```python
from build123d import *

# Parameters (mm, degrees)
SKETCH141_R  = 1.8
SKETCH141_W  = 2.5
SKETCH141_H  = 13
PAD112_DEPTH = 3


with BuildPart() as motorcageendcap:
    # Sketch141 → Pad112 (new body)
    with BuildSketch(Plane.XZ.offset(-90)):
        with BuildLine():
            Line((-29.490381, 15), (-39.5, 9.220944))
            Line((-39.5, 9.220944), (-39.5, -9.220944))
            Line((-39.5, -9.220944), (-29.490381, -15))
            Line((-24, -11.830127), (-29.490381, -15))
            Line((-24, -11.830127), (-18.128421, -22))
            Line((-18.128421, -22), (0, -22))
            Line((0, -22), (0, -19))
            ThreePointArc((0, 19), (-19, 0), (0, -19))
            Line((0, 24), (0, 19))
            Line((-16.973721, 24), (0, 24))
            Line((-24, 11.830127), (-16.973721, 24))
            Line((-29.490381, 15), (-24, 11.830127))
        make_face()
        with Locations((-29, 10)):
            Circle(SKETCH141_R, mode=Mode.SUBTRACT)
        with Locations((-29, -10)):
            Circle(SKETCH141_R, mode=Mode.SUBTRACT)
        with Locations((-12, 20)):
            Circle(SKETCH141_R, mode=Mode.SUBTRACT)
        with Locations((-36, 0)):
            Circle(SKETCH141_R, mode=Mode.SUBTRACT)
        with Locations((-30.25, 0)):
            Rectangle(SKETCH141_W, SKETCH141_H, mode=Mode.SUBTRACT)
    extrude(amount=-PAD112_DEPTH)


with BuildPart() as fusion004020018:
    # Part__Mirroring007: instance of MotorCageEndCap
    add(motorcageendcap.part.mirror(Plane(origin=(0, 0, 0), x_dir=(0, -1, 0), z_dir=(1, 0, 0))))

    # Fusion004020018: union MotorCageEndCap
    add(motorcageendcap.part)


solid = fusion004020018.part
```
Can you work these out from the model? Positions are in its coordinate system, mm. A direction names the side the tool comes from. Coordinates: 2 decimals unless noted, no trailing zeros. Loops run counter-clockwise (first coordinate to the right, second up) from the corner with the lowest first, then second, coordinate; pieces in that order, holes last. Notation, with made-up numbers: M 45.5,67.5 L 60.5,67.5 A26 ccw 60.5,100.5 Z; hole C 39,38 d7. An arc over 180 degrees is marked long. Put each result on its own line as item: value. Start each with the question number.
(1) Imagine slicing it at B-B on z = 10. List the corners of the cut face in (x, y) for me, and give its area (3 significant figures).
(2) Which directions (+Z, -Z, +X, -X, +Y, -Y) give clear straight access to the entire face, cutting with the end or side of a thin tool? Please do faces 1 (the face through (-30, 91, -6.5)), 2 (the face through (-34.43, 91.48, 12.15)), 3 (the face through (-26.784, 91.479, 13.437)), 4 (the face through (21.105, 91.479, -16.844)), 5 (the face through (-9, 93, 17)).
(3) Imagine slicing it at D-D on x = 12.5. List the corners of the cut face in (y, z) for me.
(4) Imagine slicing it at C-C on x = -8. List the corners of the cut face in (y, z) for me, and give its area (3 significant figures).
(5) I need wall thicknesses on probe 1 along Z at (x, y) = (-28, 92.85); probe 2 along X at (y, z) = (91.5, 12); probe 3 along X at (y, z) = (90.6, 3.5). Which ranges of each line are inside material? Lowest first, please.
(6) Will these pins go through, and if not, where does the flat tip stop? pin 1 Ø2 at (x, z) = (36, 0) entering from -Y; pin 2 Ø0.8 at (x, y) = (-29.5, 92) entering from -Z; pin 3 Ø1.2 at (x, y) = (30.5, 92) entering from -Z.
(7) Imagine slicing it at A-A on y = 92.15. Give the number of separate pieces and of enclosed holes in the cut face, and give its area (3 significant figures).
(8) We'd pull the mould along X, two halves only. Please class faces 6 (the face through (29, 91, 0)), 7 (the face through (0, 91, -22)), 8 (the face through (-20.536, 91.479, 17.83)), 9 (the face through (-39.5, 91, 0)): +X half, -X half, draft (parallel to the pull), parting line (faces both ways), or undercut.
Worked answers:
1. outline: M -38.15,90 L -30.8,90 L -30.8,93 L -38.15,93 Z; M -27.2,90 L -16.16,90 L -16.16,93 L -27.2,93 Z; M 16.16,90 L 27.2,90 L 27.2,93 L 16.16,93 Z; M 30.8,90 L 38.15,90 L 38.15,93 L 30.8,93 Z
1. area: 110 mm2
2. face 1: +Y, -Y
2. face 2: +Z, -X, +Y, -Y
2. face 3: +Z, +Y, -Y
2. face 4: -Z, +Y, -Y
2. face 5: +Z, -Z, +X, -X, +Y
3. outline: M 90,-22 L 93,-22 L 93,-14.31 L 90,-14.31 Z; M 90,14.31 L 93,14.31 L 93,18.27 L 90,18.27 Z; M 90,21.73 L 93,21.73 L 93,24 L 90,24 Z
4. outline: M 90,-22 L 93,-22 L 93,-17.23 L 90,-17.23 Z; M 90,17.23 L 93,17.23 L 93,24 L 90,24 Z
4. area: 34.6 mm2
5. probe 1: z = -14.14 to -11.5, -8.5 to 8.5, 11.5 to 14.14
5. probe 2: x = -34.69 to -24.29, -23.9 to -14.73, 14.73 to 23.9, 24.29 to 34.69
5. probe 3: x = -39.5 to -31.5, -29 to -18.67, 18.67 to 29, 31.5 to 39.5
6. pin 1: passes through
6. pin 2: stops at z = -15
6. pin 3: stops at z = -14.76
7. separate pieces: 1
7. enclosed holes: 11
7. area: 1,560 mm2
8. face 6: undercut
8. face 7: draft
8. face 8: undercut
8. face 9: -X half
